The model under review builds one solid part; all positions refer to its coordinate system, in mm. Face numbers are marked on the shaded views. A direction names the side the tool comes from. Coordinates: 2 decimals unless noted, no trailing zeros. Write each loop counter-clockwise with the first axis right and the second up, starting at its lowest first coordinate (ties: lowest second). Pieces come first, ordered by that corner, then holes. Notation, with made-up numbers: (78, 80) -> (104, 80) arc R16 ccw to (104, 87) -> close; hole circle Ø4 at (53.25, 64). An arc over 180 degrees is marked (long way). Write each question's results on one line, items separated by ' | '.
```python
from build123d import *

# Parameters (mm, degrees)
SKETCH1_W               = 30
SKETCH1_H               = 100
BOSS_EXTRUDE1_DEPTH     = 3.75
BOSS_EXTRUDE2_START     = -5
BOSS_EXTRUDE2_OUTLINE_W = 22.5
BOSS_EXTRUDE2_OUTLINE_H = 75
BOSS_EXTRUDE2_DEPTH     = 3


# Read off the part's stored shape, not the designer's step: Boss-Extrude2
with BuildPart() as part:
    # Sketch1 → Boss-Extrude1 (new, symmetric)
    with BuildSketch(Plane(origin=(0, 0, 0), x_dir=(1, 0, 0), z_dir=(0, 1, 0))):
        with Locations((-15, 0)):
            Rectangle(SKETCH1_W, SKETCH1_H)
    extrude(amount=BOSS_EXTRUDE1_DEPTH, both=True)

    # Boss-Extrude2 outline → Boss-Extrude2 (add)
    with BuildSketch(Plane(origin=(0, 3.75, 0), x_dir=(1, 0, 0), z_dir=(0, 1, 0)).offset(BOSS_EXTRUDE2_START)):
        with Locations((11.25, 0)):
            Rectangle(BOSS_EXTRUDE2_OUTLINE_W, BOSS_EXTRUDE2_OUTLINE_H)
    extrude(amount=BOSS_EXTRUDE2_DEPTH)


solid = part.part
```
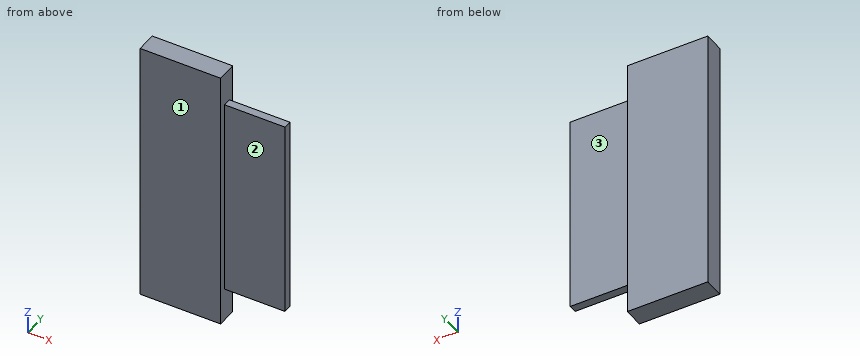
Q1. Add section C-C (x = 9). Write out the cut boundary in (y, z).
Solution:
outline: (-1.25, -37.5) -> (1.75, -37.5) -> (1.75, 37.5) -> (-1.25, 37.5) -> close
Q2. Clearance check with flat-ended pins moving along their axes: P1, Ø0.9, axis at x = 9.5, y = 0, coming from the +Z side; P2, Ø1.5, axis at x = 15.5, y = 0, coming from the -Z side; P3, Ø1.5, axis at x = 17, z = 27.5, coming from the +Y side; P4, Ø25, axis at x = 8.5, z = -5, coming from the +Y side. State where each tip first meets the part, or that it passes through.
Solution:
P1: z = 37.5 | P2: z = -37.5 | P3: y = 1.75 | P4: y = 3.75
Q3. Add section A-A (y = 0.25). Write out the cut boundary in (x, z), plus the area to 3 significant figures.
Solution:
outline: (-30, -50) -> (0, -50) -> (0, -37.5) -> (22.5, -37.5) -> (22.5, 37.5) -> (0, 37.5) -> (0, 50) -> (-30, 50) -> close | area: 4,690 mm²
Q4. Machinability: for the marked faces 1, 2 and 3, which of the approach directions +Z, -Z, +X, -X, +Y, -Y give a long, thin tool a straight path to every point of the face, cutting with its end or side? Answer none if there is none.
Solution:
face 1: +Z, -Z, +X, -X, -Y | face 2: +Z, -Z, +X, -Y | face 3: +Z, -Z, +X, +Y
Q5. Add section B-B (z = -16.5). Write out the cut boundary in (x, y), plus the area to 4 significant figures.
Solution:
outline: (-30, -3.75) -> (0, -3.75) -> (0, -1.25) -> (22.5, -1.25) -> (22.5, 1.75) -> (0, 1.75) -> (0, 3.75) -> (-30, 3.75) -> close | area: 292.5 mm²
Q6. For line 1 (X direction, y = 3.5, z = -24.5); line 2 (Y direction, x = 16, z = -28), list the stretches that pass through material, from the lowest coordinate up. Write a range as from..to.
Solution:
line 1: -30..0 | line 2: -1.25..1.75
